from build123d import *

# Parameters (mm, degrees)
SKETCH1_R           = 9
SKETCH1_R_2         = 1.55
BOSS_EXTRUDE1_DEPTH = 1.9
SKETCH2_R           = 3
BOSS_EXTRUDE2_DEPTH = 1.5
SKETCH3_R           = 2.5
BOSS_EXTRUDE3_DEPTH = 2.4
SKETCH4_R           = 2.95
CUT_EXTRUDE1_DEPTH  = 0.6
CHAMFER1_SIZE       = 1.4


with BuildPart() as part:
    # Sketch1 → Boss-Extrude1 (new body)
    with BuildSketch(Plane(origin=(0, 0, 0), x_dir=(0, 1, 0), z_dir=(0, 0, 1))):
        with Locations(Location((0, 0, 0), (0, 0, 90))):
            Circle(SKETCH1_R)
        with Locations(Location((-4.242640687, 4.242640687, 0), (0, 0, 90))):
            Circle(SKETCH1_R_2, mode=Mode.SUBTRACT)
        with Locations(Location((4.242640687, 4.242640687, 0), (0, 0, 90))):
            Circle(SKETCH1_R_2, mode=Mode.SUBTRACT)
        with Locations(Location((4.242640687, -4.242640687, 0), (0, 0, 90))):
            Circle(SKETCH1_R_2, mode=Mode.SUBTRACT)
        with Locations(Location((-4.242640687, -4.242640687, 0), (0, 0, 90))):
            Circle(SKETCH1_R_2, mode=Mode.SUBTRACT)
    extrude(amount=BOSS_EXTRUDE1_DEPTH)

    # Sketch2 → Boss-Extrude2 (add)
    with BuildSketch(Plane.XY.offset(1.9)):
        Circle(SKETCH2_R)
    extrude(amount=BOSS_EXTRUDE2_DEPTH)

    # Sketch3 → Boss-Extrude3 (add)
    with BuildSketch(Plane.XY.offset(3.4)):
        Circle(SKETCH3_R)
    extrude(amount=BOSS_EXTRUDE3_DEPTH)

    # Sketch4 → Cut-Extrude1 (cut)
    with BuildSketch(Plane.XY.offset(1.9)):
        with Locations((-4.242640687, 4.242640687)):
            Circle(SKETCH4_R)
        with Locations((4.242640687, 4.242640687)):
            Circle(SKETCH4_R)
        with Locations((4.242640687, -4.242640687)):
            Circle(SKETCH4_R)
        with Locations((-4.242640687, -4.242640687)):
            Circle(SKETCH4_R)
    extrude(amount=-CUT_EXTRUDE1_DEPTH, mode=Mode.SUBTRACT)

    # Chamfer1
    # the kernel refuses this chamfer: 1.4 mm, written as the material it takes off along each edge
    with BuildSketch(Plane(origin=(-4.242640687, -4.242640687, 1.3), x_dir=(-1, 0, 0), z_dir=(0, -1, 0))) as chamfer1_piece_1_section:
        Polygon((1.55, CHAMFER1_SIZE), (1.55 + CHAMFER1_SIZE, 0), (1.55, 0), align=None)
    chamfer1_piece_1 = revolve(axis=Axis((-4.242640687, -4.242640687, 1.3), (0, 0, -1)), mode=Mode.PRIVATE)
    chamfer1_piece_1 = chamfer1_piece_1 & Plane(origin=(-4.242640687, -4.242640687, 0.597078296), x_dir=(1, 0, 0), z_dir=(0, 0, 1)) * Cylinder(2.95, 12, mode=Mode.PRIVATE)
    add(chamfer1_piece_1, mode=Mode.SUBTRACT)
    with BuildSketch(Plane(origin=(4.242640687, -4.242640687, 1.3), x_dir=(-1, 0, 0), z_dir=(0, -1, 0))) as chamfer1_piece_2_section:
        Polygon((1.55, CHAMFER1_SIZE), (1.55 + CHAMFER1_SIZE, 0), (1.55, 0), align=None)
    chamfer1_piece_2 = revolve(axis=Axis((4.242640687, -4.242640687, 1.3), (0, 0, -1)), mode=Mode.PRIVATE)
    chamfer1_piece_2 = chamfer1_piece_2 & Plane(origin=(4.242640687, -4.242640687, 0.597078296), x_dir=(1, 0, 0), z_dir=(0, 0, 1)) * Cylinder(2.95, 12, mode=Mode.PRIVATE)
    add(chamfer1_piece_2, mode=Mode.SUBTRACT)
    with BuildSketch(Plane(origin=(4.242640687, 4.242640687, 1.3), x_dir=(-1, 0, 0), z_dir=(0, -1, 0))) as chamfer1_piece_3_section:
        Polygon((1.55, CHAMFER1_SIZE), (1.55 + CHAMFER1_SIZE, 0), (1.55, 0), align=None)
    chamfer1_piece_3 = revolve(axis=Axis((4.242640687, 4.242640687, 1.3), (0, 0, -1)), mode=Mode.PRIVATE)
    chamfer1_piece_3 = chamfer1_piece_3 & Plane(origin=(4.242640687, 4.242640687, 0.597078296), x_dir=(1, 0, 0), z_dir=(0, 0, 1)) * Cylinder(2.95, 12, mode=Mode.PRIVATE)
    add(chamfer1_piece_3, mode=Mode.SUBTRACT)
    with BuildSketch(Plane(origin=(-4.242640687, 4.242640687, 1.3), x_dir=(-1, 0, 0), z_dir=(0, -1, 0))) as chamfer1_piece_4_section:
        Polygon((1.55, CHAMFER1_SIZE), (1.55 + CHAMFER1_SIZE, 0), (1.55, 0), align=None)
    chamfer1_piece_4 = revolve(axis=Axis((-4.242640687, 4.242640687, 1.3), (0, 0, -1)), mode=Mode.PRIVATE)
    chamfer1_piece_4 = chamfer1_piece_4 & Plane(origin=(-4.242640687, 4.242640687, 0.597078296), x_dir=(1, 0, 0), z_dir=(0, 0, 1)) * Cylinder(2.95, 12, mode=Mode.PRIVATE)
    add(chamfer1_piece_4, mode=Mode.SUBTRACT)


solid = part.part
Design review of the part built by this model. Coordinates are the model's own, in mm. A direction names the side the tool comes from. Coordinates: 2 decimals unless noted, no trailing zeros. Order: outer loops, then holes, each group sorted by start corner. A loop starts at its lowest first (then second) coordinate and runs counter-clockwise, first axis right, second up.
Item 1: For pin 1 Ø3.5 at (x, y) = (-4.24, 4.24) entering from +Z, flat-tipped, find the tip position at first contact; note if it passes through.
Item 2: The part is to be moulded in two halves that separate along X. For faces 1 (the cylindrical face through (-1.429, -3.357, 1.604)), 2 (the cylindrical face through (-0.54, -2.44, 4.58)), 3 (the flat face through (0, 0, 0)), 4 (the cylindrical face through (3.859, 7.168, 1.604)), say which applies: pulls with the +X half, pulls with the -X half, needs draft (parallel to the pull), parting line crosses it, or undercut.
Item 3: Take a section at A-A, the plane x = 0. Write out the cut boundary in (y, z).
Item 4: For line 1 (Y direction, x = 5.5, z = 1.2) (3 decimals); line 2 (X direction, y = 3.75, z = 1.2); line 3 (Y direction, x = -1.75, z = 1.15), list the stretches that pass through material, from the lowest coordinate up.
Item 5: Take a section at D-D, the plane y = -5.5. Count the separate pieces of the cut face and the enclosed holes in it, then the cut area to 3 significant figures.
Item 6: Take a section at C-C, the plane z = 2.6. Write out the cut boundary in (x, y).
Item 7: For faces 5 (the cylindrical face through (-8.584, -2.703, 0.937)), 6 (the cylindrical face through (7.056, -3.357, 1.604)), list the 3-axis set-ups (+Z, -Z, +X, -X, +Y, -Y) from which the entire face can be reached by the end or side of a thin tool; tool diameter is ignored.
The answers:
1. pin 1: stops at z = 0.1
2. face 1: undercut
2. face 2: parting line crosses it
2. face 3: needs draft
2. face 4: undercut
3. outline: (-9, 0) - (9, 0) - (9, 1.9) - (3, 1.9) - (3, 3.4) - (2.5, 3.4) - (2.5, 5.8) - (-2.5, 5.8) - (-2.5, 3.4) - (-3, 3.4) - (-3, 1.9) - (-9, 1.9) - close
4. line 1: y = -7.124 to -6.8, -1.685 to 1.685, 6.8 to 7.124
4. line 2: x = -8.18 to -7.05, -1.44 to 1.44, 7.05 to 8.18
4. line 3: y = -8.83 to -5.52, -2.97 to 2.97, 5.52 to 8.83
5. separate pieces: 3
5. enclosed holes: 0
5. area: 10.7 mm2
6. outline: circle Ø6 at (0, 0)
7. face 5: +Z, -Z
7. face 6: +Z
